Geometry: final body of the model. Coordinates: model frame, mm. Face numbers are marked on the shaded views. A direction names the side the tool comes from. Coordinates: 2 decimals unless noted, no trailing zeros. Order: outer loops, then holes, each group sorted by start corner. A loop starts at its lowest first (then second) coordinate and runs counter-clockwise, first axis right, second up. Notation, with made-up numbers: M 71,17.25 L 80,17.25 A20 cw 80,29.25 Z; hole C 73,34.25 d8. An arc over 180 degrees is marked long. Use CSV: the item, a comma, the result in double quotes. Start each with the question number.
Q1. First-contact query: P1, Ø2, axis at x = -2, y = 1.5, coming from the +Z side; P2, Ø2, axis at x = 0, z = 4, coming from the +Y side; P3, Ø1.5, axis at x = -4.5, y = 4, coming from the -Z side. Flat tips, straight axial feed; report the tip coordinate or a pass-through.
Q2. Section query D-D, the plane y = 2.5. Output: boundary loops of the cut face in (x, z).
Q3. Section query C-C, the plane y = -7. Output: boundary loops of the cut face in (x, z) (3 decimals), and give its area (3 significant figures).
Q4. Section query B-B, the plane x = -1.5. Output: boundary loops of the cut face in (y, z) (3 decimals), and give its area (4 significant figures).
Q5. Mould query, pull axis X, two halves, no side actions, for the marked faces 3, 4 and 5. Classes: +X half, -X half, draft (parallel to the pull), parting line (faces both ways), or undercut.
Q6. Section query A-A, the plane z = 4.75. Output: boundary loops of the cut face in (x, y) (3 decimals).
Q7. Ray query, probe 1 along Y at (x, z) = (-7, 2.8) (3 decimals); probe 2 along Z at (x, y) = (-2.75, 0.5); probe 3 along X at (y, z) = (-1.5, 4.1). Return the intervals inside material, ascending.
Q8. Access query for the marked faces 1 and 2. Directions: +Z, -Z, +X, -X, +Y, -Y. A direction counts if a zero-diameter tool reaches every point of the face in a straight line with its end or side. Return the directions, or none.
from build123d import *

# Parameters (mm, degrees)
SKETCH_1_W              = 5
SKETCH_1_H              = 20
EXTRUDE_1_DEPTH         = 5
SKETCH1_W               = 5
SKETCH1_H               = 20
EXTRUDE1_DEPTH          = 6.8
M2_5_TAPPED_HOLE1_D     = 2.05
M2_5_TAPPED_HOLE1_DEPTH = 6.35
M2_5_TAPPED_HOLE1_TIP   = 0.615882135
EXTRUDE2_DEPTH          = 2.5
SKETCH3_W               = 11.8
SKETCH3_H               = 3.5
EXTRUDE3_DEPTH          = 5
SKETCH4_W               = 5
SKETCH4_H               = 5
EXTRUDE4_DEPTH          = 2.5
CHAMFER4_SIZE           = 2
SKETCH8_W               = 2
SKETCH8_H               = 5
EXTRUDE6_DEPTH          = 2.5
FILLET1_R               = 0.5
FILLET2_R               = 0.5
CHAMFER6_SIZE           = 3.5
CHAMFER6_SIZE2          = 6.062177826
SKETCH12_W              = 5
SKETCH12_H              = 16.5
EXTRUDE11_DEPTH         = 0.5
EXTRUDE10_REACH         = 21.357
CHAMFER9_SIZE           = 1
FILLET3_R               = 5


with BuildPart() as part:
    # 草图1 → 拉伸1 (new body)
    with BuildSketch(Plane.XY):
        Rectangle(SKETCH_1_W, SKETCH_1_H)
    extrude(amount=EXTRUDE_1_DEPTH)

    # Sketch1 → Extrude1 (add)
    with BuildSketch(Plane.ZY.offset(2.5)):
        with Locations((2.5, 0)):
            Rectangle(SKETCH1_W, SKETCH1_H)
    extrude(amount=EXTRUDE1_DEPTH)

    # M2.5 Tapped Hole1
    with Locations(Plane(origin=(-1.5, -7, 0), x_dir=(-1, 0, 0), z_dir=(0, 0, -1))):
        with Locations((0, 0), (5.5, 5)):
            Hole(M2_5_TAPPED_HOLE1_D / 2, depth=M2_5_TAPPED_HOLE1_DEPTH)
            with Locations((0, 0, -(M2_5_TAPPED_HOLE1_DEPTH + M2_5_TAPPED_HOLE1_TIP / 2))):  # 118° drill point
                Cone(0, M2_5_TAPPED_HOLE1_D / 2, M2_5_TAPPED_HOLE1_TIP, mode=Mode.SUBTRACT)

    # Sketch2 → Extrude2 (cut)
    with BuildSketch(Plane(origin=(0, 0, 5), x_dir=(-1, 0, 0), z_dir=(0, 0, -1))):
        with BuildLine():
            Line((-1.5, -1.7), (-1.5, 5.5))
            ThreePointArc((-1.5, 5.5), (-1.207106781, 6.207106781), (-0.5, 6.5))
            Line((-0.5, 6.5), (2.5, 6.5))
            ThreePointArc((2.5, 6.5), (3.207106781, 6.207106781), (3.5, 5.5))
            Line((3.5, 5.5), (3.5, -1.7))
            ThreePointArc((3.5, -1.7), (3.207106781, -2.407106781), (2.5, -2.7))
            Line((2.5, -2.7), (-0.5, -2.7))
            ThreePointArc((-0.5, -2.7), (-1.207106781, -2.407106781), (-1.5, -1.7))
        make_face()
    extrude(amount=EXTRUDE2_DEPTH, mode=Mode.SUBTRACT)

    # Sketch3 → Extrude3 (cut)
    with BuildSketch(Plane.XY.offset(5)):
        with Locations((-3.4, 8.25)):
            Rectangle(SKETCH3_W, SKETCH3_H)
    extrude(amount=-EXTRUDE3_DEPTH, mode=Mode.SUBTRACT)

    # Sketch4 → Extrude4 (cut)
    with BuildSketch(Plane(origin=(0, 0, 5), x_dir=(-1, 0, 0), z_dir=(0, 0, -1))):
        with Locations((1, 5.5)):
            Rectangle(SKETCH4_W, SKETCH4_H)
    extrude(amount=EXTRUDE4_DEPTH, mode=Mode.SUBTRACT)

    # Chamfer4
    chamfer4_edges = [part.edges().sort_by_distance(p)[0] for p in [
        (2.5, -1.75, 0),
    ]]
    chamfer(chamfer4_edges, length=CHAMFER4_SIZE)

    # Sketch8 → Extrude6 (cut)
    with BuildSketch(Plane.XY.offset(5)):
        with Locations((1.5, -0.2)):
            Rectangle(SKETCH8_W, SKETCH8_H)
    extrude(amount=-EXTRUDE6_DEPTH, mode=Mode.SUBTRACT)

    # Fillet1
    fillet1_edges = [part.edges().sort_by_distance(p)[0] for p in [
        (1.5, 2.3, 3.75),
    ]]
    fillet(fillet1_edges, radius=FILLET1_R)

    # Fillet2
    fillet2_edges = [part.edges().sort_by_distance(p)[0] for p in [
        (-3.5, 6.5, 3.75),
        (1.5, 6.5, 3.75),
    ]]
    fillet(fillet2_edges, radius=FILLET2_R)

    # Chamfer6
    chamfer6_edges = [part.edges().sort_by_distance(p)[0] for p in [
        (2.5, -10, 3.5),
    ]]
    chamfer6_side = [part.faces().sort_by_distance(p)[0] for p in [
        (-3.583625731, -10, 2.564327485),
    ]]
    chamfer(chamfer6_edges, length=CHAMFER6_SIZE, length2=CHAMFER6_SIZE2, reference=chamfer6_side[0])

    # Sketch12 → Extrude11 (cut)
    with BuildSketch(Plane.ZY.offset(9.3)):
        with Locations((2.5, -1.75)):
            Rectangle(SKETCH12_W, SKETCH12_H)
    extrude(amount=-EXTRUDE11_DEPTH, mode=Mode.SUBTRACT)

    # Extrude10: up to this face of the body (flat: up to its plane)
    extrude10_end = Plane(part.part.faces().sort_by_distance((-4.9, -10, 2.5))[0])
    # Sketch13 → Extrude10 (cut, up to the picked face)
    with BuildSketch(Plane(origin=(0, 6.5, 0), x_dir=(1, 0, 0), z_dir=(0, 1, 0)), mode=Mode.PRIVATE) as extrude10_sk1:
        Polygon((-8.8, -3), (-8.8, 0), (-3.603847577, 0), align=None)
    extrude10_tool1 = split(extrude(extrude10_sk1.sketch, amount=-EXTRUDE10_REACH, mode=Mode.PRIVATE), bisect_by=extrude10_end, keep=Keep.BOTH, mode=Mode.PRIVATE)
    add(extrude10_tool1.solids().sort_by(Axis((-7.067949, 6.5, 1), (0, -1, 0)))[0], mode=Mode.SUBTRACT)

    # Chamfer9
    chamfer9_edges = [part.edges().sort_by_distance(p)[0] for p in [
        (-8.8, 6.5, 4),
        (-8.8, -10, 4),
    ]]
    chamfer(chamfer9_edges, length=CHAMFER9_SIZE)

    # Fillet3
    fillet3_edges = [part.edges().sort_by_distance(p)[0] for p in [
        (2.5, -3.937822174, 3.5),
    ]]
    fillet(fillet3_edges, radius=FILLET3_R)


solid = part.part
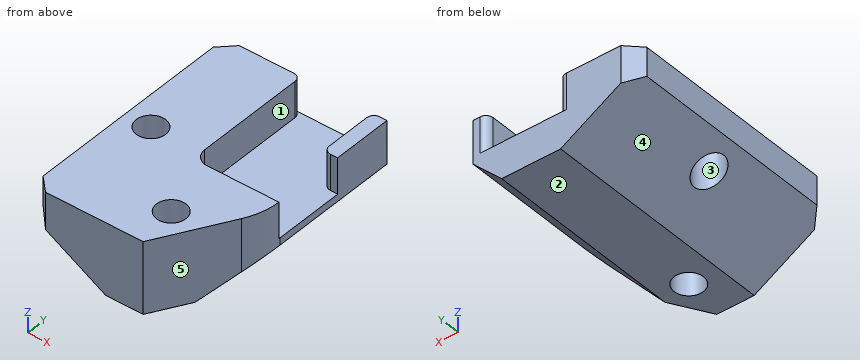
Responses:
1,P1,"stops at z = 2.5"
1,P2,"stops at y = -2.7"
1,P3,"stops at z = 0.08"
2,outline,"M -8.8,3 L -3.6,0 L 0.5,0 L 2.5,2 L 2.5,5 L 1.6,5 L 1.6,2.5 L -3.5,2.5 L -3.5,5 L -8.8,5 Z"
3,outline,"M -8.8,3 L -3.604,0 L -2.525,0 L -2.525,5 L -8.8,5 Z; M -0.475,0 L 0.5,0 L 0.732,0.232 L 0.732,5 L -0.475,5 Z"
3,area,"29.6 mm²"
4,outline,"M -10,0 L -8.025,0 L -8.025,5 L -10,5 Z; M -5.975,0 L 6.5,0 L 6.5,2.5 L -2.7,2.5 L -2.7,5 L -5.975,5 Z"
4,area,"49.25 mm²"
5,face 3,"undercut"
5,face 4,"-X half"
5,face 5,"+X half"
6,outline,"M -8.8,-9 L -7.8,-10 L -1,-10 L 1.83,-5.098 A5 ccw 2.499,-2.7 L -2.5,-2.7 A1 cw -3.5,-1.7 L -3.5,6 A0.5 ccw -4,6.5 L -7.8,6.5 L -8.8,5.5 Z; M 1.5,2.8 A0.5 ccw 2,2.3 L 2.5,2.3 L 2.5,6.5 L 2,6.5 A0.5 ccw 1.5,6 Z; hole C -7,-2 d2.05; hole C -1.5,-7 d2.05"
7,probe 1,"y = -10 to -3.025, -0.975 to 6.5"
7,probe 2,"z = 0 to 2.5"
7,probe 3,"x = -8.8 to -7.89, -6.11 to -3.5"
8,face 1,"+Z, +Y"
8,face 2,"-Z, +X, -X, +Y, -Y"
